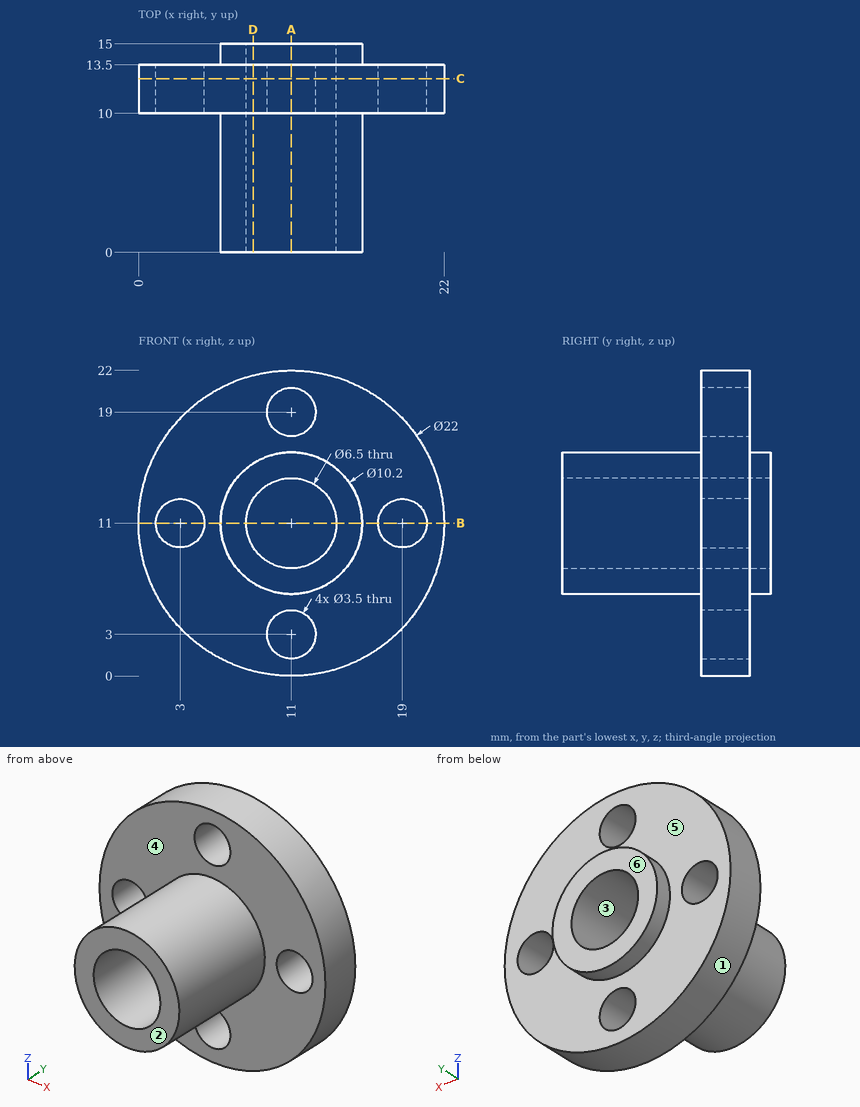
Could you check a few things on this drawing? It's one solid part, dimensions in mm from its lowest x, y, z. A direction names the side the tool comes from. Give positions to 0.01 mm unless a question says otherwise; leave off trailing zeros. Loops run counter-clockwise (first coordinate to the right, second up) from the corner with the lowest first, then second, coordinate; pieces in that order, holes last. Notation, with made-up numbers: M -39,-33.5 L -8,-33.5 A36 cw -8,4.5 Z; hole C 73.5,-8.5 d3. An arc over 180 degrees is marked long. One line per question, with ' | ' between items. Start each with the question number.
Q1. If we section it at A-A (x = 11): Please give me the cut outline in (y, z).
Q2. If we mould it in two halves opening along X, with no side actions, what happens to the marked faces 1, 2 and 3? For each: +X half, -X half, draft (parallel to the pull), parting line (faces both ways), or undercut.
Q3. If we section it at D-D (x = 8.25): Please give me the cut outline in (y, z).
Q4. For pin 1 Ø4 at (x, z) = (10, 18.5) entering from -Y; pin 2 Ø1.5 at (y, z) = (4, 5) entering from -X; pin 3 Ø8 at (x, z) = (5.5, 8) entering from +Y; pin 4 Ø5 at (y, z) = (12.5, 17.5) entering from +X, each with a flat end and sliding along its axis, tell me the tip position at first contact or that it passes through.
Q5. If we section it at B-B (z = 11): Please give me the cut outline in (x, y), plus the area to 3 significant figures.
Q6. If I drill on line 1 (X direction, y = 11.35, z = 11); line 2 (X direction, y = 5.5, z = 11); line 3 (Y direction, x = 6.75, z = 20.5), over which ranges is the centre line in solid material (lowest first)? Write a range as from..to.
Q7. If we section it at C-C (y = 12.5): Please give me the cut outline in (x, z).
Q8. For the marked faces 4, 5 and 6, which set-ups out of +Z, -Z, +X, -X, +Y, -Y let a thin tool reach every point of the face, with its end or its side?
Computed:
1) outline: M 0,5.9 L 10,5.9 L 10,4.75 L 13.5,4.75 L 13.5,5.9 L 15,5.9 L 15,7.75 L 0,7.75 Z; M 0,14.25 L 15,14.25 L 15,16.1 L 13.5,16.1 L 13.5,17.25 L 10,17.25 L 10,16.1 L 0,16.1 Z; M 10,0 L 13.5,0 L 13.5,1.25 L 10,1.25 Z; M 10,20.75 L 13.5,20.75 L 13.5,22 L 10,22 Z
2) face 1: parting line | face 2: draft | face 3: undercut
3) outline: M 0,6.7 L 10,6.7 L 10,0.35 L 13.5,0.35 L 13.5,6.7 L 15,6.7 L 15,9.27 L 0,9.27 Z; M 0,12.73 L 15,12.73 L 15,15.3 L 13.5,15.3 L 13.5,21.65 L 10,21.65 L 10,15.3 L 0,15.3 Z
4) pin 1: stops at y = 10 | pin 2: passes through | pin 3: stops at y = 15 | pin 4: stops at x = 21.25
5) outline: M 0,10 L 1.25,10 L 1.25,13.5 L 0,13.5 Z; M 4.75,10 L 5.9,10 L 5.9,0 L 7.75,0 L 7.75,15 L 5.9,15 L 5.9,13.5 L 4.75,13.5 Z; M 14.25,0 L 16.1,0 L 16.1,10 L 17.25,10 L 17.25,13.5 L 16.1,13.5 L 16.1,15 L 14.25,15 Z; M 20.75,10 L 22,10 L 22,13.5 L 20.75,13.5 Z | area: 72.3 mm²
6) line 1: x = 0..1.25, 4.75..7.75, 14.25..17.25, 20.75..22 | line 2: x = 5.9..7.75, 14.25..16.1 | line 3: y = 10..13.5
7) outline: C 11,11 d22; hole C 3,11 d3.5; hole C 11,11 d6.5; hole C 11,3 d3.5; hole C 11,19 d3.5; hole C 19,11 d3.5
8) face 4: -Y | face 5: +Y | face 6: +Z, -Z, +X, -X, +Y
